from build123d import *

# Parameters (mm, degrees)
F0_W     = 50.8
F0_H     = 25.4
F1_DEPTH = 12.7
F2_R     = 12.7
F3_DEPTH = 25.4
F4_R     = 6.35
F5_DEPTH = 25.4
F7_DEPTH = 12.7


with BuildPart() as f1:
    # F0 (on Top) → F1 (new body)
    with BuildSketch(Plane.XY):
        with Locations((-18.8566240436, 44.6426421404)):
            Rectangle(F0_W, F0_H)
        with BuildLine():
            Line((-44.2566240436, 31.9426421404), (-44.2566240436, 57.3426421404))
            ThreePointArc((-44.2566240436, 57.3426421404), (-56.9566240436, 44.6426421404), (-44.2566240436, 31.9426421404))
        make_face()
        with BuildLine():
            ThreePointArc((6.5433759564, 31.9426421404), (19.2433759564, 44.6426421404), (6.5433759564, 57.3426421404))
            Line((6.5433759564, 57.3426421404), (6.5433759564, 31.9426421404))
        make_face()
    extrude(amount=F1_DEPTH)

    # F2 (on face) → F3 (join)
    with BuildSketch(Plane.XY.offset(12.7)):
        with Locations((-44.2566240436, 44.6426421404)):
            Circle(F2_R)
    extrude(amount=F3_DEPTH)

    # F4 (on face) → F5 (cut)
    with BuildSketch(Plane.XY.offset(38.1)):
        with Locations((-44.2566240436, 44.6426421404)):
            Circle(F4_R)
    extrude(amount=-F5_DEPTH, mode=Mode.SUBTRACT)

    # F6 (on face) → F7 (cut)
    with BuildSketch(Plane.XY.offset(12.7)):
        with BuildLine():
            ThreePointArc((7.0575587453, 38.3134940097), (11.2117568701, 40.3381422106), (12.8933759564, 44.6426421404))
            ThreePointArc((12.8933759564, 44.6426421404), (11.2117568701, 48.9471420701), (7.0575587453, 50.971790271))
            Line((7.0575587453, 50.971790271), (7.0575587453, 38.3134940097))
        make_face()
        with BuildLine():
            Line((6.0291931675, 50.971790271), (7.0575587453, 50.971790271))
            ThreePointArc((7.0575587453, 50.971790271), (6.5433759564, 50.9926421404), (6.0291931675, 50.971790271))
        make_face()
        with BuildLine():
            Line((7.0575587453, 38.3134940097), (7.0575587453, 50.971790271))
            Line((7.0575587453, 50.971790271), (6.0291931675, 50.971790271))
            ThreePointArc((6.0291931675, 50.971790271), (0.1933759564, 44.6426421404), (6.0291931675, 38.3134940097))
            Line((6.0291931675, 38.3134940097), (7.0575587453, 38.3134940097))
        make_face()
        with BuildLine():
            ThreePointArc((6.0291931675, 38.3134940097), (6.5433759564, 38.2926421404), (7.0575587453, 38.3134940097))
            Line((7.0575587453, 38.3134940097), (6.0291931675, 38.3134940097))
        make_face()
        with BuildLine():
            ThreePointArc((6.0291931675, 38.3134940097), (0.1933759564, 44.6426421404), (6.0291931675, 50.971790271))
            Line((6.0291931675, 50.971790271), (-18.3424412547, 50.971790271))
            ThreePointArc((-18.3424412547, 50.971790271), (-14.1882431299, 48.9471420701), (-12.5066240436, 44.6426421404))
            ThreePointArc((-12.5066240436, 44.6426421404), (-14.1882431299, 40.3381422106), (-18.3424412547, 38.3134940097))
            Line((-18.3424412547, 38.3134940097), (6.0291931675, 38.3134940097))
        make_face()
        with BuildLine():
            Line((-18.3424412547, 38.3134940097), (-18.3424412547, 50.971790271))
            ThreePointArc((-18.3424412547, 50.971790271), (-25.2066240436, 44.6426421404), (-18.3424412547, 38.3134940097))
        make_face()
        with BuildLine():
            ThreePointArc((-12.5066240436, 44.6426421404), (-14.1882431299, 48.9471420701), (-18.3424412547, 50.971790271))
            Line((-18.3424412547, 50.971790271), (-18.3424412547, 38.3134940097))
            ThreePointArc((-18.3424412547, 38.3134940097), (-14.1882431299, 40.3381422106), (-12.5066240436, 44.6426421404))
        make_face()
    extrude(amount=-F7_DEPTH, mode=Mode.SUBTRACT)


solid = f1.part
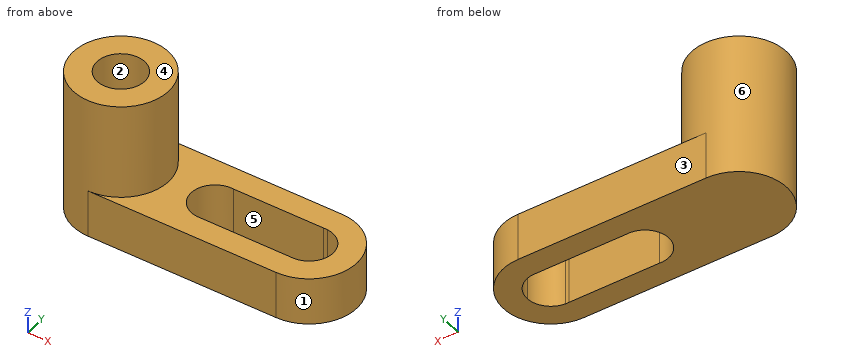
Geometry: final body of the model. Coordinates: model frame, mm. Face numbers are marked on the shaded views. A direction names the side the tool comes from. Give positions to 0.01 mm unless a question says otherwise; leave off trailing zeros. Loops run counter-clockwise (first coordinate to the right, second up) from the corner with the lowest first, then second, coordinate; pieces in that order, holes last. Notation, with made-up numbers: M 68.25,15.25 L 74.25,15.25 A21 cw 74.25,19.25 Z; hole C 51.25,41.5 d9. An arc over 180 degrees is marked long. Put each result on its own line as item: value. Start each with the question number.
1) Contact query for flat-ended pins moving along their axis: pin 1 (7.5 mm diameter, centred on x = -26, y = 49.5, fed in from +Z); pin 2 (6 mm diameter, centred on y = 50.5, z = 25, fed in from -X); pin 3 (2 mm diameter, centred on y = 51.5, z = 13.5, fed in from +X). Output: stop coordinate, or through.
2) Access query for the marked faces 4, 5 and 6. Directions: +Z, -Z, +X, -X, +Y, -Y. A direction counts if a zero-diameter tool reaches every point of the face in a straight line with its end or side. Return the directions, or none.
3) Pull-direction query (X, two-part tool) for the marked faces 1, 2 and 3; classes: pulls with the +X half, pulls with the -X half, needs draft (parallel to the pull), parting line crosses it, or undercut.
4) Cut plane B-B (y = 49). Output: boundary loops of the cut face in (x, z).
5) Cut plane D-D (x = -43). Output: boundary loops of the cut face in (y, z), then the cut area to 3 significant figures.
6) Ray query, line 1 along Y through (x, z) = (3.5, 7); line 2 along X through (y, z) = (45.75, 21) (3 decimals); line 3 along X through (y, z) = (42.75, 8.5). Return the intervals inside material, ascending.
7) Cut plane A-A (x = 5). Output: boundary loops of the cut face in (y, z).
8) Cut plane C-C (z = 31). Output: boundary loops of the cut face in (x, y), then the cut area to 3 significant figures.
Verdict:
1. pin 1: z = 12.7
1. pin 2: x = -56.63
1. pin 3: x = 17.59
2. face 4: +Z, +X, -X, +Y, -Y
2. face 5: +Z, -Z
2. face 6: +Z
3. face 1: pulls with the +X half
3. face 2: undercut
3. face 3: needs draft
4. outline: M -56.19,0 L -23.48,0 L -23.48,12.7 L -32.33,12.7 L -32.33,38.1 L -39.64,38.1 L -39.64,12.7 L -48.88,12.7 L -48.88,38.1 L -56.19,38.1 Z; M 11.16,0 L 18.47,0 L 18.47,12.7 L 11.16,12.7 Z
5. outline: M 31.94,0 L 57.34,0 L 57.34,12.7 L 57.28,12.7 L 57.28,38.1 L 50.87,38.1 L 50.87,12.7 L 38.42,12.7 L 38.42,38.1 L 32,38.1 L 32,12.7 L 31.94,12.7 Z
5. area: 648 mm2
6. line 1: 31.94 to 38.31, 50.97 to 57.34
6. line 2: -56.908 to -50.509, -38.004 to -31.605
6. line 3: -56.81 to -24.92, 12.6 to 19.1
7. outline: M 31.94,0 L 38.31,0 L 38.31,12.7 L 31.94,12.7 Z; M 50.97,0 L 57.34,0 L 57.34,12.7 L 50.97,12.7 Z
8. outline: C -44.26,44.64 d25.4; hole C -44.26,44.64 d12.7
8. area: 380 mm2
